Source: three-view drawing plus pictorial views. Frame: mm from the lowest corner of the part. Coordinates: 2 decimals unless noted, no trailing zeros. Write each loop counter-clockwise with the first axis right and the second up, starting at its lowest first coordinate (ties: lowest second). Pieces come first, ordered by that corner, then holes. Notation, with made-up numbers: (40, -28.5) -> (60, -28.5) arc R23 cw to (60, -7.5) -> close; hole circle Ø4 at (54, 84). An arc over 180 degrees is marked (long way). One line per item, written item: value.
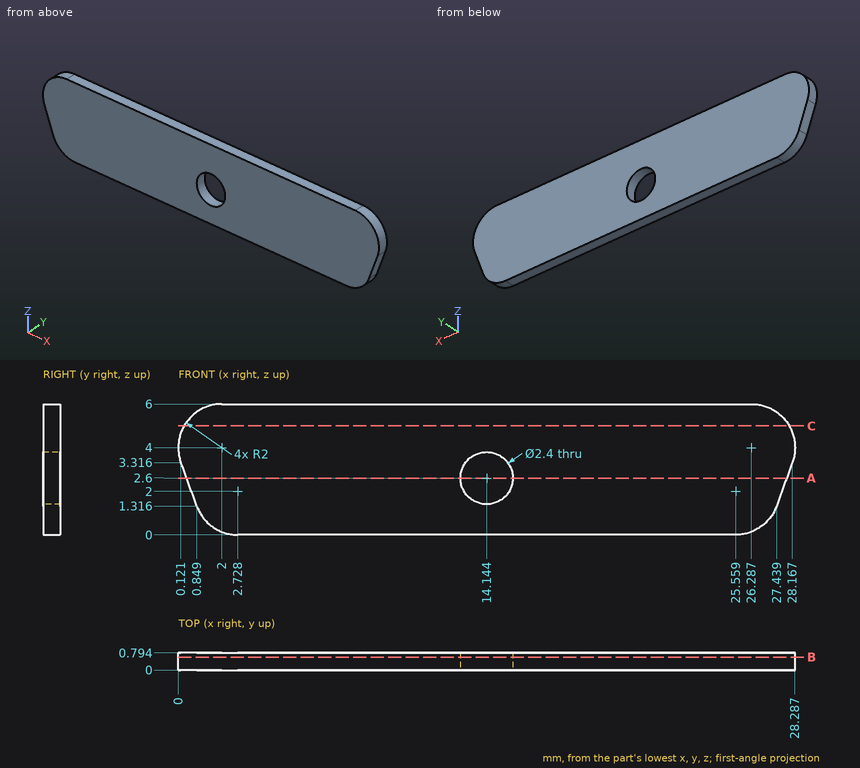
(1) Line query: line 1 (Z direction, x = 14.25, y = 0.55) (1 decimal); line 2 (X direction, y = 0.4, z = 2.6) (1 decimal); line 3 (X direction, y = 0.7, z = 1.6) (1 decimal). Output: solid intervals per line, ascending. Write a range as [from, to].
Responses:
line 1: z = [0, 1.4], [3.8, 6]
line 2: x = [0.4, 12.9], [15.3, 27.9]
line 3: x = [0.7, 13.5], [14.8, 27.5]
(2) Section A-A (z = 2.6). Return the cut outline in (x, y).
Responses:
outline: (0.38, 0) -> (12.94, 0) -> (12.94, 0.79) -> (0.38, 0.79) -> close; (15.34, 0) -> (27.91, 0) -> (27.91, 0.79) -> (15.34, 0.79) -> close
(3) Section C-C (z = 5). Return the cut outline in (x, y).
Responses:
outline: (0.27, 0) -> (28.02, 0) -> (28.02, 0.79) -> (0.27, 0.79) -> close
(4) Section B-B (y = 0.6). Return the cut outline in (x, z), then the cut area to 3 significant figures.
Responses:
outline: (0.12, 3.32) -> (0.85, 1.32) arc R2 ccw to (2.73, 0) -> (25.56, 0) arc R2 ccw to (27.44, 1.32) -> (28.17, 3.32) arc R2 ccw to (26.29, 6) -> (2, 6) arc R2 ccw to start; hole circle Ø2.4 at (14.14, 2.6)
area: 158 mm2
